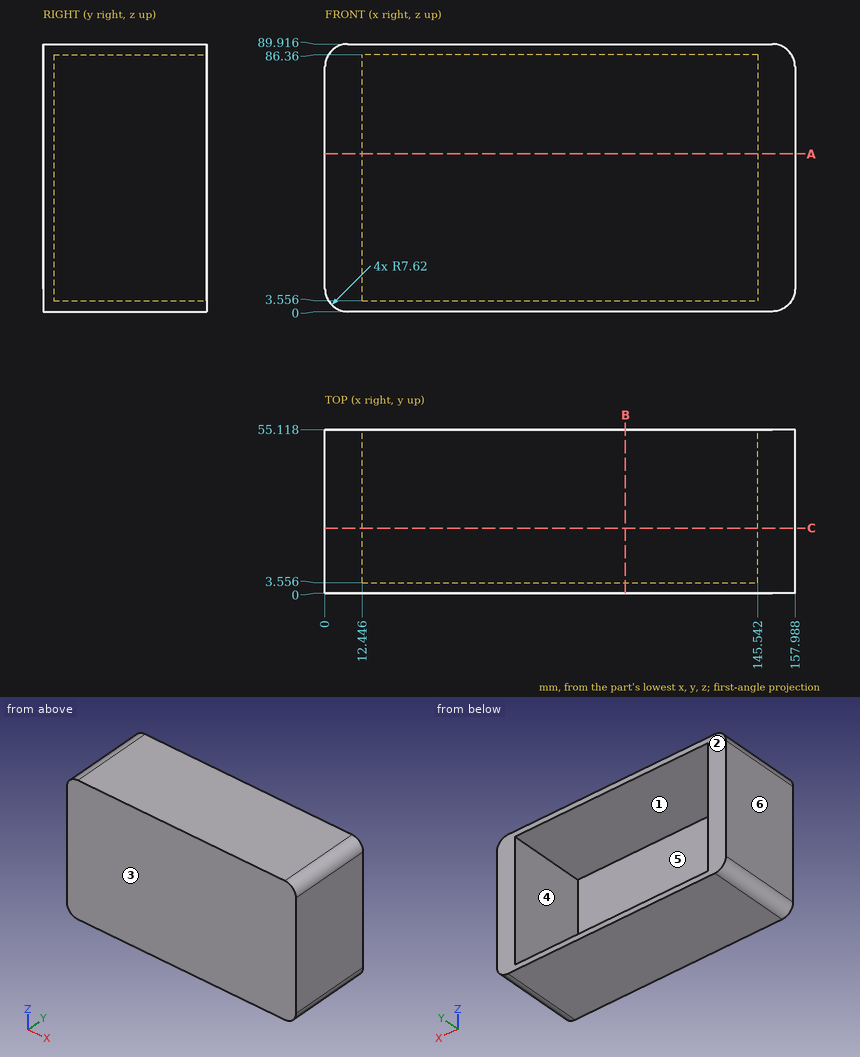
Part print with two shaded views. Sizes in mm from the minimum x, y, z corner. A direction names the side the tool comes from. Coordinates: 2 decimals unless noted, no trailing zeros. Order: outer loops, then holes, each group sorted by start corner. A loop starts at its lowest first (then second) coordinate and runs counter-clockwise, first axis right, second up.
(1) Drill centre lines: L1, parallel to X at y = 25.5, z = 39; L2, parallel to Z at x = 39.5, y = 5; L3, parallel to Y at x = 74.5, z = 35.5. Where is each one in solid material? Low to high.
Solution:
L1: x = 0 to 12.45, 145.54 to 157.99
L2: z = 0 to 3.56, 86.36 to 89.92
L3: y = 0 to 3.56
(2) Which spindle directions (+Z, -Z, +X, -X, +Y, -Y) get a long thin tool onto all of the face, cutting with end or side? Do the marked faces 1 and 2. Say none if no direction does.
Solution:
face 1: +Y
face 2: +Z, -Z, +X, -X, +Y
(3) Saw through at C-C, the plane y = 22. Write the cut outline in (x, z).
Solution:
outline: (0, 7.62) arc R7.62 ccw to (7.62, 0) - (150.37, 0) arc R7.62 ccw to (157.99, 7.62) - (157.99, 82.3) arc R7.62 ccw to (150.37, 89.92) - (7.62, 89.92) arc R7.62 ccw to (0, 82.3) - close; hole (12.45, 3.56) - (145.54, 3.56) - (145.54, 86.36) - (12.45, 86.36) - close
(4) Saw through at A-A, the plane z = 53. Write the cut outline in (x, y), and give its area (3 significant figures).
Solution:
outline: (0, 0) - (157.99, 0) - (157.99, 55.12) - (145.54, 55.12) - (145.54, 3.56) - (12.45, 3.56) - (12.45, 55.12) - (0, 55.12) - close
area: 1,850 mm2
(5) Pin check, flat tip, straight feed: pin 1 Ø2 at (x, z) = (96, 16) entering from +Y. Stop position of the tip, or through.
Solution:
pin 1: stops at y = 3.56
(6) Mould opens along X. For the marked faces 3, 4, 5 and 6 say: released by +X, released by -X, zero draft, split by the parting line, or undercut.
Solution:
face 3: zero draft
face 4: undercut
face 5: undercut
face 6: released by -X
(7) Saw through at B-B, the plane x = 101. Write the cut outline in (y, z), and give its area (3 significant figures).
Solution:
outline: (0, 0) - (55.12, 0) - (55.12, 3.56) - (3.56, 3.56) - (3.56, 86.36) - (55.12, 86.36) - (55.12, 89.92) - (0, 89.92) - close
area: 686 mm2
